Could you check a few things on this drawing? It's one solid part, dimensions in mm from its lowest x, y, z. A direction names the side the tool comes from. Coordinates: 2 decimals unless noted, no trailing zeros. Order: outer loops, then holes, each group sorted by start corner. A loop starts at its lowest first (then second) coordinate and runs counter-clockwise, first axis right, second up.
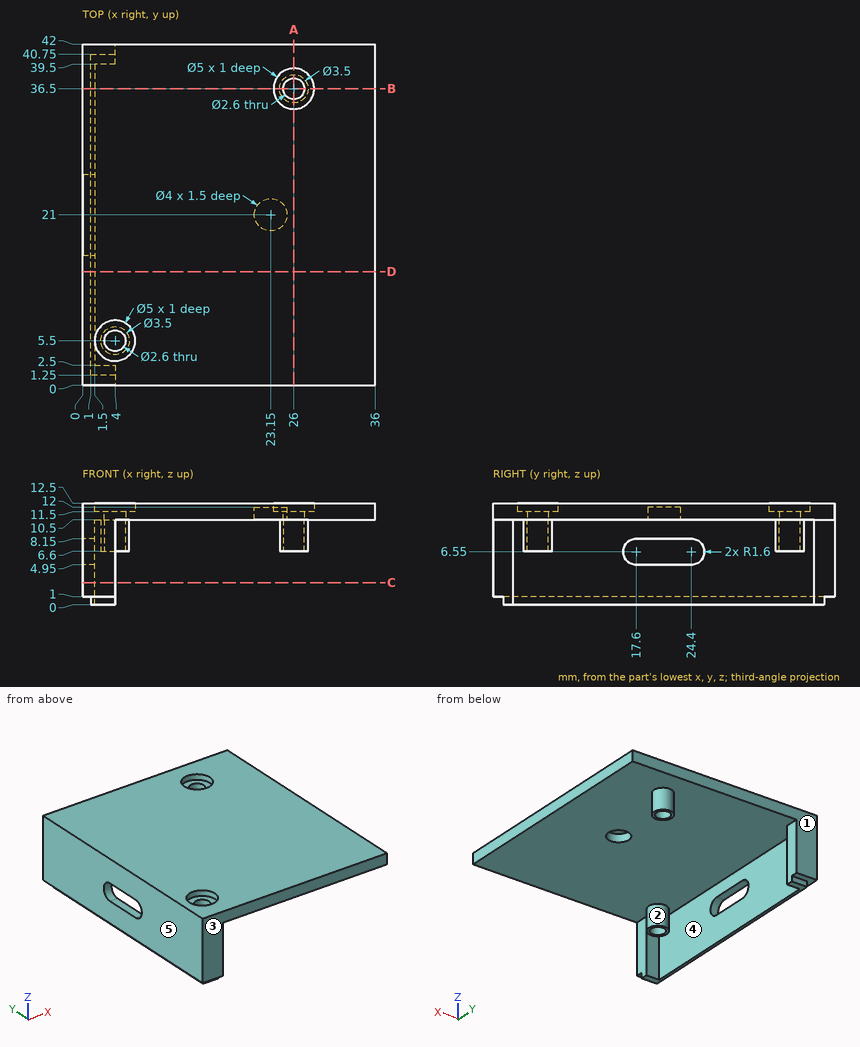
Q1. I need wall thicknesses on L1, parallel to Y at x = 26, z = 8.85; L2, parallel to Y at x = 26, z = 12; L3, parallel to X at y = 36.5, z = 11. Which ranges of each line are inside material? Lowest first, please.
Q2. Will these pins go through, and if not, where does the flat tip stop? pin 1 (3 mm diameter, centred on x = 4, y = 5.5, fed in from -Z); pin 2 (2 mm diameter, centred on x = 16, y = 9, fed in from -Z); pin 3 (0.5 mm diameter, centred on x = 3, z = 0.5, fed in from -Y).
Q3. If we section it at C-C on z = 2.75: Write out the boundary of the cut face in (x, y).
Q4. If we section it at B-B on y = 36.5: Write out the boundary of the cut face in (x, z).
Q5. For the marked faces 1 and 2, which set-ups out of +Z, -Z, +X, -X, +Y, -Y let a thin tool reach every point of the face, with its end or its side?
Q6. If we section it at D-D on y = 14: Write out the boundary of the cut face in (x, z), then the cut area to 4 significant figures.
Q7. If we section it at A-A on x = 26: Write out the boundary of the cut face in (y, z).
Q8. We'd pull the mould along Y, two halves only. Please class the marked faces 3, 4 and 5: pulls with the +Y half, pulls with the -Y half, needs draft (parallel to the pull), parting line crosses it, or undercut.
Reply:
1. L1: y = 34.75 to 35.2, 37.8 to 38.25
1. L2: y = 0 to 34, 39 to 42
1. L3: x = 0 to 24.7, 27.3 to 36
2. pin 1: stops at z = 6.6
2. pin 2: stops at z = 10.5
2. pin 3: stops at y = 1.25
3. outline: (0, 0) - (4, 0) - (4, 2.5) - (1.5, 2.5) - (1.5, 39.5) - (4, 39.5) - (4, 42) - (0, 42) - close
4. outline: (0, 1) - (1, 1) - (1, 0) - (1.5, 0) - (1.5, 10.5) - (24.25, 10.5) - (24.25, 6.6) - (24.7, 6.6) - (24.7, 11.5) - (23.5, 11.5) - (23.5, 12.5) - (0, 12.5) - close; (27.3, 6.6) - (27.75, 6.6) - (27.75, 10.5) - (36, 10.5) - (36, 12.5) - (28.5, 12.5) - (28.5, 11.5) - (27.3, 11.5) - close
5. face 1: +Z, -Z, +X, -X, +Y
5. face 2: -Z
6. outline: (0, 1) - (1, 1) - (1, 0) - (1.5, 0) - (1.5, 10.5) - (36, 10.5) - (36, 12.5) - (0, 12.5) - close
6. area: 86.75 mm2
7. outline: (0, 10.5) - (34.75, 10.5) - (34.75, 6.6) - (35.2, 6.6) - (35.2, 11.5) - (34, 11.5) - (34, 12.5) - (0, 12.5) - close; (37.8, 6.6) - (38.25, 6.6) - (38.25, 10.5) - (42, 10.5) - (42, 12.5) - (39, 12.5) - (39, 11.5) - (37.8, 11.5) - close
8. face 3: pulls with the -Y half
8. face 4: undercut
8. face 5: needs draft
